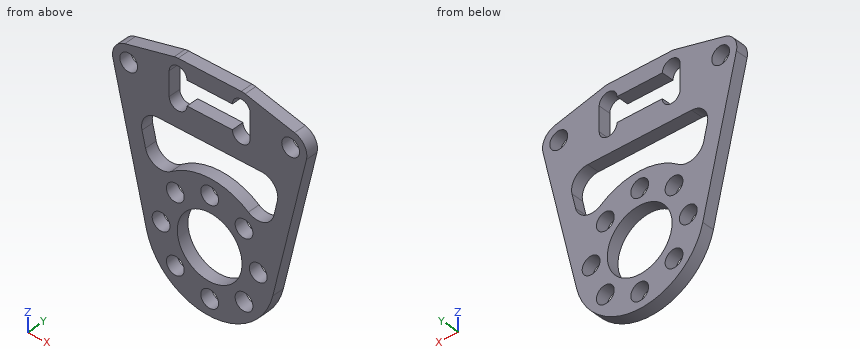
Autodesk Inventor part; units mm, degrees
ref_plane "YZ Plane" through (0, 0, 0) normal (1, 0, 0) x (0, 1, 0)
ref_plane "XZ Plane" through (0, 0, 0) normal (0, 1, 0) x (-1, 0, 0)
ref_plane "XY Plane" through (0, 0, 0) normal (0, 0, 1) x (1, 0, 0)
sketch "スケッチ1" plane through (0, 0, 0) normal (0, 1, 0) x (-1, 0, 0)
  circle A0 centre (0, 0) radius 4
  circle A1 centre (0, 0) radius 6 construction
  circle A2 centre (0, 0) radius 8
  circle A3 centre (0, -6) radius 1.1
  circle A4 centre (4.2426, -4.2426) radius 1.1
  circle A5 centre (6, 0) radius 1.1
  circle A6 centre (4.2426, 4.2426) radius 1.1
  circle A7 centre (0, 6) radius 1.1
  circle A8 centre (-4.2426, 4.2426) radius 1.1
  circle A9 centre (-6, 0) radius 1.1
  circle A10 centre (-4.2426, -4.2426) radius 1.1
  line L0 (5, 15) -> (-5, 15)
  line L1 (-5, 15) -> (-5, 18)
  line L2 (-5, 18) -> (5, 18)
  line L3 (5, 18) -> (5, 15)
  circle A11 centre (3.9, 15) radius 1.1
  line L4 (0, 15) -> (0, 18) construction
  circle A12 centre (-3.9, 15) radius 1.1
  line L5 (-5, 16.5) -> (5, 16.5) construction
  circle A13 centre (3.9, 18) radius 1.1
  circle A14 centre (-3.9, 18) radius 1.1
  circle A15 centre (-10, 16.5) radius 1.1
  circle A16 centre (10, 16.5) radius 1.1
  circle A17 centre (10, 16.5) radius 2
  circle A18 centre (3.9, 18) radius 2
  circle A19 centre (-10, 16.5) radius 2
  line L6 (7.7918, -1.8132) -> (11.948, 16.0467)
  line L7 (-7.7918, -1.8132) -> (-11.948, 16.0467)
  line L8 (10.4776, 18.4421) -> (4.3776, 19.9421)
  circle A20 centre (-3.9, 18) radius 2
  line L9 (-10.4776, 18.4421) -> (-4.3776, 19.9421)
  line L10 (3.9, 20) -> (-4.1423, 20)
  point P0 (2.8, 18)
  point P1 (5, 18)
  point P2 (2.8, 15)
  point P3 (-2.8, 15)
  point P4 (-5, 15)
  point P5 (-5, 18)
  point P6 (-2.8, 18)
  point P7 (-3.9, 20)
  point P8 (-10.4776, 18.4421)
  dimension "d1" = 12
  dimension "d11" = 2.2
  dimension "d16" = 4
  dimension "d0" = 8
  dimension "d2" = 16
  dimension "d3" = 2.2
  dimension "d6" = 360
  dimension "d8" = 10
  dimension "d9" = 3
  dimension "d10" = 15
  dimension "d12" = 2.2
  dimension "d13" = 5
  dimension "d14" = 4
  dimension "d15" = 4
extrude "押し出し1" add sketch "スケッチ1" along normal blind 1.5 contours A2 | A2 L7 A19 L9 A20 L1 A12 L0 A11 L3 A18 L8 A17 L6 | A19 | A17 | A20 L2 A14 L1 | A18 L3 A13 L2 | L10 A18 L2 A20
sketch "スケッチ2" plane through (0, 1.5, 0) normal (0, 1, 0) x (1, 0, 0)
  line L0 (-8.9295, -11.9) -> (8.9295, -11.9)
  line L1 (8.9295, -11.9) -> (7.0432, -3.7939)
  line L2 (-7.7918, 1.8132) -> (-11.948, -16.0467)
  circle A0 centre (0, 0) radius 8
  line L3 (-8.9295, -11.9) -> (-7.0432, -3.7939)
  line L4 (-7.7918, 1.8132) -> (-11.948, -16.0467)
  line L5 (11.948, -16.0467) -> (7.7918, 1.8132)
  arc A1 (-2.8, -15) -> (-5, -15) centre (-3.9, -15) ccw
  point P0 (-3.9, -13.9)
  dimension "d19" = 2
  dimension "d20" = 2
  dimension "d21" = 2
extrude "押し出し2" cut sketch "スケッチ2" against normal through all contours L3 A0 L1 L0
fillet "フィレット1" radius 2 4 edges at (-7.0432, 0.75, 3.7939) (7.0432, 0.75, 3.7939) (8.9295, 0.75, 11.9) (-8.9295, 0.75, 11.9)
equation "\"d21\" = d19"
properties part number "kata" material "アルミニウム 2014-T4"
Verification items for the finished model (mm, model axes). Give positions to 0.01 mm unless a question says otherwise; leave off trailing zeros. Loops run counter-clockwise (first coordinate to the right, second up) from the corner with the lowest first, then second, coordinate; pieces in that order, holes last.
1. Cross-section at D-D on x = -10. Record the cut outline in (y, z).
Derived:
outline: (0, 7.68) - (1.5, 7.68) - (1.5, 15.4) - (0, 15.4) - close; (0, 17.6) - (1.5, 17.6) - (1.5, 18.56) - (0, 18.56) - close
2. Cross-section at B-B on z = 3.5. Record the cut outline in (x, y), and give its area (3 significant figures).
Derived:
outline: (-9.03, 0) - (-5.05, 0) - (-5.05, 1.5) - (-9.03, 1.5) - close; (-3.43, 0) - (-1.94, 0) - (-1.94, 1.5) - (-3.43, 1.5) - close; (1.94, 0) - (3.43, 0) - (3.43, 1.5) - (1.94, 1.5) - close; (5.05, 0) - (9.03, 0) - (9.03, 1.5) - (5.05, 1.5) - close
area: 16.4 mm2
3. Cross-section at C-C on z = 8.5. Record the cut outline in (x, y).
Derived:
outline: (-10.19, 0) - (-8.14, 0) - (-8.14, 1.5) - (-10.19, 1.5) - close; (8.14, 0) - (10.19, 0) - (10.19, 1.5) - (8.14, 1.5) - close
4. Material ranges on probe 1 along X at (y, z) = (0.25, 4.75); probe 2 along X at (y, z) = (0.8, -0.25); probe 3 along X at (y, z) = (1.2, 1), recorded low to high.
Derived:
probe 1: x = -9.32 to -5.22, -3.27 to 3.27, 5.22 to 9.32
probe 2: x = -8.16 to -7.07, -4.93 to -3.99, 3.99 to 4.93, 7.07 to 8.16
probe 3: x = -8.45 to -6.46, -5.54 to -3.87, 3.87 to 5.54, 6.46 to 8.45
5. Go/stop test with flat-tipped pins: P1, Ø2, axis at x = 0, z = 6, coming from the +Y side; P2, Ø0.8, axis at y = 0.5, z = 17, coming from the -X side. Record where each tip stops, or that it passes through.
Derived:
P1: passes through
P2: stops at x = -12
6. Cross-section at A-A on x = 0. Record the cut outline in (y, z).
Derived:
outline: (0, -8) - (1.5, -8) - (1.5, -7.1) - (0, -7.1) - close; (0, -4.9) - (1.5, -4.9) - (1.5, -4) - (0, -4) - close; (0, 4) - (1.5, 4) - (1.5, 4.9) - (0, 4.9) - close; (0, 7.1) - (1.5, 7.1) - (1.5, 8) - (0, 8) - close; (0, 11.9) - (1.5, 11.9) - (1.5, 15) - (0, 15) - close; (0, 18) - (1.5, 18) - (1.5, 20) - (0, 20) - close
